from build123d import *

# Parameters (mm, degrees)
SALIENTE_EXTRUIR1_DEPTH = 100
CROQUIS2_R              = 6
CORTAR_EXTRUIR1_DEPTH   = 100


with BuildPart() as part:
    # Croquis1 → Saliente-Extruir1 (new body)
    with BuildSketch(Plane.XY):
        with BuildLine():
            Line((8, -8), (8, -120))
            Line((8, -120), (-8, -120))
            Line((-8, -120), (-8, -8))
            ThreePointArc((-8, -8), (-3.313708499, 3.313708499), (8, 8))
            Line((8, 8), (100, 8))
            Line((100, 8), (100, -8))
            Line((100, -8), (8, -8))
        make_face()
    extrude(amount=SALIENTE_EXTRUIR1_DEPTH)

    # Croquis2 → Cortar-Extruir1 (cut)
    with BuildSketch(Plane(origin=(8, 0, 0), x_dir=(0, 0, -1), z_dir=(1, 0, 0))):
        with Locations((-84.666164139, -28.683062658)):
            Circle(CROQUIS2_R)
        with Locations((-48.336024121, -28.683062658)):
            Circle(CROQUIS2_R)
        with Locations((-15.333835861, -28.683062658)):
            Circle(CROQUIS2_R)
        with Locations((-74.682308867, -99.956696128)):
            Circle(CROQUIS2_R)
        with Locations((-30.309618769, -99.956696128)):
            Circle(CROQUIS2_R)
    extrude(amount=-CORTAR_EXTRUIR1_DEPTH, mode=Mode.SUBTRACT)


solid = part.part
Geometry: final body of the model. Coordinates: model frame, mm. A direction names the side the tool comes from. Round coordinates to 2 decimals unless told otherwise and drop trailing zeros. Loops run counter-clockwise (first coordinate to the right, second up) from the corner with the lowest first, then second, coordinate; pieces in that order, holes last.
Q1. Section C-C on y = -25. Return loops of the section in (x, z), plus the area to 3 significant figures.
Q2. Pin query (flat end, axial travel): P1, Ø2, axis at x = 87, z = 35, coming from the -Y side; P2, Ø19, axis at y = -28.68, z = 15.33, coming from the +X side. Return the tip coordinate at first contact, or that it passes through.
Q3. Section B-B on z = 67. Return loops of the section in (x, y), plus the area to 3 significant figures.
Q4. Section D-D on x = 50. Return loops of the section in (y, z), plus the area to 3 significant figures.
Q5. Section A-A on z = 34.5. Return loops of the section in (x, y).
Q6. Pull-direction query (Y, two-part tool) for faces 1 (the flat face through (55, -8, 49)), 2 (the cylindrical face through (0.112, -34.006, 45.567)), 3 (the flat face through (6, -32, 0)); classes: released by +Y, released by -Y, zero draft, split by the parting line, or undercut.
Q7. Material intervals for L1, parallel to X at y = -112.5, z = 84.5; L2, parallel to Y at x = 7.5, z = 94.5, sorted ascending.
Q8. Access query for faces 4 (the flat face through (8, -63, 49)), 5 (the cylindrical face through (-3.437, 3.189, 49.3)). Directions: +Z, -Z, +X, -X, +Y, -Y. A direction counts if a zero-diameter tool reaches every point of the face in a straight line with its end or side. Return the directions, or none.
Evaluation:
1. outline: (-8, 0) - (8, 0) - (8, 10.6) - (-8, 10.6) - close; (-8, 20.07) - (8, 20.07) - (8, 43.6) - (-8, 43.6) - close; (-8, 53.07) - (8, 53.07) - (8, 79.93) - (-8, 79.93) - close; (-8, 89.4) - (8, 89.4) - (8, 100) - (-8, 100) - close
1. area: 1,150 mm2
2. P1: stops at y = -8
2. P2: stops at x = 8
3. outline: (-8, -120) - (8, -120) - (8, -8) - (100, -8) - (100, 8) - (8, 8) arc R16 ccw to (-8, -8) - close
3. area: 3,470 mm2
4. outline: (-8, 0) - (8, 0) - (8, 100) - (-8, 100) - close
4. area: 1,600 mm2
5. outline: (-8, -120) - (8, -120) - (8, -104.25) - (-8, -104.25) - close; (-8, -95.66) - (8, -95.66) - (8, -8) - (100, -8) - (100, 8) - (8, 8) arc R16 ccw to (-8, -8) - close
6. face 1: released by -Y
6. face 2: undercut
6. face 3: zero draft
7. L1: x = -8 to 8
7. L2: y = -120 to 7.99
8. face 4: +Z, -Z, +X, -Y
8. face 5: +Z, -Z, -X, +Y
